Verification items for the finished model (mm, model axes). Face numbers are marked on the shaded views. A direction names the side the tool comes from. Coordinates: 2 decimals unless noted, no trailing zeros. Order: outer loops, then holes, each group sorted by start corner. A loop starts at its lowest first (then second) coordinate and runs counter-clockwise, first axis right, second up. Notation, with made-up numbers: (-35, 68.25) -> (-25, 68.25) arc R11 ccw to (-25, 86.25) -> close; hole circle Ø11 at (46, 17). An arc over 180 degrees is marked (long way). Answer as CSV lines item,"result".
```python
from build123d import *

# Parameters (mm, degrees)
BOSS_EXTRUDE1_DEPTH = 50.8
FILLET1_R           = 0.762


with BuildPart() as part:
    # Sketch1 → Boss-Extrude1 (new body)
    with BuildSketch(Plane.XY):
        with BuildLine():
            Line((0.921, -2.954280738), (0.921, -1.524))
            ThreePointArc((0.921, -1.524), (2.101945458, 1.327054542), (4.953, 2.508))
            Line((4.953, 2.508), (11.053129195, 2.508))
            ThreePointArc((11.053129195, 2.508), (11.884634671, 3.434294742), (13.081, 3.778))
            Line((13.081, 3.778), (25.019, 3.778))
            ThreePointArc((25.019, 3.778), (26.215365329, 3.434294742), (27.046870805, 2.508))
            Line((27.046870805, 2.508), (47.830933704, 2.508))
            ThreePointArc((47.830933704, 2.508), (49.356721017, 2.431266869), (50.867111376, 2.201841804))
            ThreePointArc((50.867111376, 2.201841804), (54.276645107, 0.167640195), (55.671506067, -3.549517234))
            Line((55.671506067, -3.549517234), (55.671506067, -18.802482766))
            ThreePointArc((55.671506067, -18.802482766), (54.276645107, -22.519640195), (50.867111376, -24.553841804))
            ThreePointArc((50.867111376, -24.553841804), (49.356721017, -24.783266869), (47.830933704, -24.86))
            Line((47.830933704, -24.86), (4.953, -24.86))
            ThreePointArc((4.953, -24.86), (2.101945458, -23.679054542), (0.921, -20.828))
            Line((0.921, -20.828), (0.921, -19.397719262))
            ThreePointArc((0.921, -19.397719262), (-1.509208506, -18.333027258), (-2.508, -15.875))
            Line((-2.508, -15.875), (-2.508, -6.477))
            ThreePointArc((-2.508, -6.477), (-1.509208506, -4.018972742), (0.921, -2.954280738))
        make_face()
        with BuildLine():
            Line((12.954, 0.889), (12.954, 1.143))
            ThreePointArc((12.954, 1.143), (13.102789755, 1.502210245), (13.462, 1.651))
            Line((13.462, 1.651), (24.638, 1.651))
            ThreePointArc((24.638, 1.651), (24.997210245, 1.502210245), (25.146, 1.143))
            Line((25.146, 1.143), (25.146, 0.889))
            ThreePointArc((25.146, 0.889), (25.294789755, 0.529789755), (25.654, 0.381))
            Line((25.654, 0.381), (47.830933704, 0.381))
            ThreePointArc((47.830933704, 0.381), (49.143323488, 0.314998811), (50.442469746, 0.117661273))
            ThreePointArc((50.442469746, 0.117661273), (52.637548133, -1.187962697), (53.544506067, -3.575524294))
            Line((53.544506067, -3.575524294), (53.544506067, -18.776475706))
            ThreePointArc((53.544506067, -18.776475706), (52.637548133, -21.164037303), (50.442469746, -22.469661273))
            ThreePointArc((50.442469746, -22.469661273), (49.143323488, -22.666998811), (47.830933704, -22.733))
            Line((47.830933704, -22.733), (4.953, -22.733))
            ThreePointArc((4.953, -22.733), (3.605961582, -22.175038418), (3.048, -20.828))
            Line((3.048, -20.828), (3.048, -17.907))
            ThreePointArc((3.048, -17.907), (2.862012806, -17.457987194), (2.413, -17.272))
            Line((2.413, -17.272), (1.016, -17.272))
            ThreePointArc((1.016, -17.272), (0.028171827, -16.862828173), (-0.381, -15.875))
            Line((-0.381, -15.875), (-0.381, -6.477))
            ThreePointArc((-0.381, -6.477), (0.028171827, -5.489171827), (1.016, -5.08))
            Line((1.016, -5.08), (2.413, -5.08))
            ThreePointArc((2.413, -5.08), (2.862012806, -4.894012806), (3.048, -4.445))
            Line((3.048, -4.445), (3.048, -1.524))
            ThreePointArc((3.048, -1.524), (3.605961582, -0.176961582), (4.953, 0.381))
            Line((4.953, 0.381), (12.446, 0.381))
            ThreePointArc((12.446, 0.381), (12.805210245, 0.529789755), (12.954, 0.889))
        make_face(mode=Mode.SUBTRACT)
    extrude(amount=BOSS_EXTRUDE1_DEPTH)

    # Fillet1
    fillet1_edges = [part.edges().sort_by_distance(p)[0] for p in [
        (0.921, -2.954280738, 25.4),
        (0.921, -19.397719262, 25.4),
        (27.046870805, 2.508, 25.4),
        (11.053129195, 2.508, 25.4),
    ]]
    fillet(fillet1_edges, radius=FILLET1_R)


solid = part.part
```
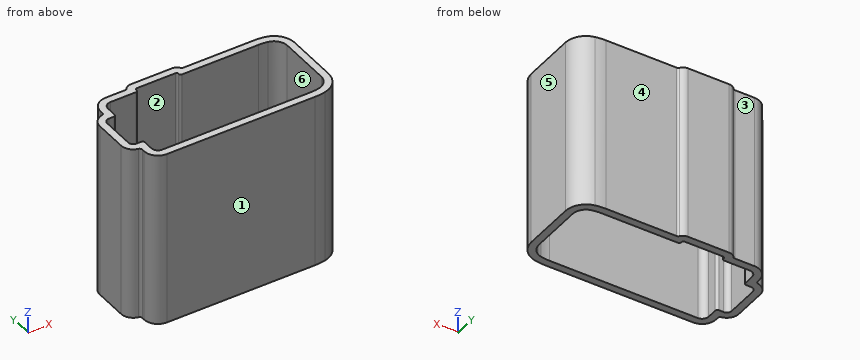
Item 1: Thickness scan on line 1 (Y direction, x = 10.5, z = 14.5); line 2 (Y direction, x = 16, z = 7); line 3 (X direction, y = -11.5, z = 29). Record the ranges inside material, lowest first.
Answer list:
line 1,"-24.86 to -22.73, 0.38 to 2.51"
line 2,"-24.86 to -22.73, 1.65 to 3.78"
line 3,"-2.51 to -0.38, 53.54 to 55.67"
Item 2: Release check for a two-part mould opening along Y. For the marked faces 1, 2 and 3 record: +Y half, -Y half, draft (parallel to the pull), parting line (faces both ways), or undercut.
Answer list:
face 1,"-Y half"
face 2,"undercut"
face 3,"+Y half"
Item 3: Section check A-A, the plane y = -9. Record the boundary of the cut face in (x, z).
Answer list:
outline,"(-2.51, 0) -> (-0.38, 0) -> (-0.38, 50.8) -> (-2.51, 50.8) -> close; (53.54, 0) -> (55.67, 0) -> (55.67, 50.8) -> (53.54, 50.8) -> close"
Item 4: Section check B-B, the plane x = 36. Record the boundary of the cut face in (y, z), plus the area to 3 significant figures.
Answer list:
outline,"(-24.86, 0) -> (-22.73, 0) -> (-22.73, 50.8) -> (-24.86, 50.8) -> close; (0.38, 0) -> (2.51, 0) -> (2.51, 50.8) -> (0.38, 50.8) -> close"
area,"216 mm2"
Item 5: Tool access check on the marked faces 4, 5 and 6. Record the directions out of +Z, -Z, +X, -X, +Y, -Y that give a thin tool (end or side, any length) a straight path to the whole face; none if there is none.
Answer list:
face 4,"+Z, -Z, +X, +Y"
face 5,"+Z, -Z, +X, +Y, -Y"
face 6,"+Z, -Z"
Item 6: Depth check by flat-ended pin: pin 1 Ø1.5 at (y, z) = (-2.5, 27.5) entering from +X; pin 2 Ø0.8 at (y, z) = (-2, 28) entering from -X; pin 3 Ø3 at (x, z) = (9, 26.5) entering from +Y. Enter the tip coordinate at first touch or a pass-through.
Answer list:
pin 1,"x = 55.66"
pin 2,"x = 0.91"
pin 3,"y = 2.51"
